Geometry check sheet. Reference: the model listing, model coordinates, mm. Give positions to 0.01 mm unless a question says otherwise; leave off trailing zeros. Write each loop counter-clockwise with the first axis right and the second up, starting at its lowest first coordinate (ties: lowest second). Pieces come first, ordered by that corner, then holes. Notation, with made-up numbers: (80, 69) -> (108, 69) arc R21 ccw to (108, 77) -> close; hole circle Ø10 at (80, -10.5). An arc over 180 degrees is marked (long way). One line per item, written item: value.
from build123d import *

# Parameters (mm, degrees)
F0_W     = 175
F0_H     = 130
F0_R     = 7.5
F1_DEPTH = 15


with BuildPart() as f1:
    # F0 (on Front) → F1 (new body)
    with BuildSketch(Plane.XZ):
        Rectangle(F0_W, F0_H)
        with Locations((-62.5, -40)):
            Circle(F0_R, mode=Mode.SUBTRACT)
        with Locations((-37.5, -40)):
            Circle(F0_R, mode=Mode.SUBTRACT)
        with Locations((-12.5, -40)):
            Circle(F0_R, mode=Mode.SUBTRACT)
        with Locations((12.5, -40)):
            Circle(F0_R, mode=Mode.SUBTRACT)
        with Locations((37.5, -40)):
            Circle(F0_R, mode=Mode.SUBTRACT)
        with Locations((62.5, -40)):
            Circle(F0_R, mode=Mode.SUBTRACT)
        with Locations((-62.5, 0)):
            Circle(F0_R, mode=Mode.SUBTRACT)
        with Locations((-37.5, 0)):
            Circle(F0_R, mode=Mode.SUBTRACT)
        with Locations((-12.5, 0)):
            Circle(F0_R, mode=Mode.SUBTRACT)
        with Locations((-62.5, 40)):
            Circle(F0_R, mode=Mode.SUBTRACT)
        with Locations((-37.5, 40)):
            Circle(F0_R, mode=Mode.SUBTRACT)
        with Locations((-12.5, 40)):
            Circle(F0_R, mode=Mode.SUBTRACT)
        with Locations((12.5, 0)):
            Circle(F0_R, mode=Mode.SUBTRACT)
        with Locations((37.5, 0)):
            Circle(F0_R, mode=Mode.SUBTRACT)
        with Locations((62.5, 0)):
            Circle(F0_R, mode=Mode.SUBTRACT)
        with Locations((12.5, 40)):
            Circle(F0_R, mode=Mode.SUBTRACT)
        with Locations((37.5, 40)):
            Circle(F0_R, mode=Mode.SUBTRACT)
        with Locations((62.5, 40)):
            Circle(F0_R, mode=Mode.SUBTRACT)
    extrude(amount=F1_DEPTH)


solid = f1.part
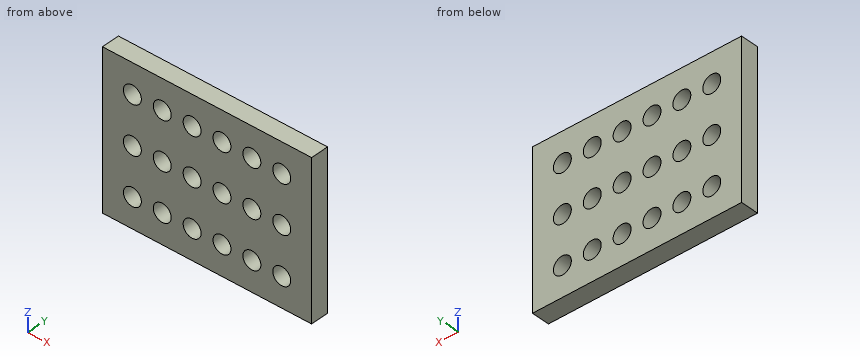
1) Scan lines: probe 1 along Z at (x, y) = (37.5, -4.5); probe 2 along Z at (x, y) = (14.5, -11). Record each from-to range of solid material in increasing order.
Verdict:
probe 1: -65 to -47.5, -32.5 to -7.5, 7.5 to 32.5, 47.5 to 65
probe 2: -65 to -47.23, -32.77 to -7.23, 7.23 to 32.77, 47.23 to 65
2) Sectioned sample at B-B on x = -62.5. Record the cut outline in (y, z), plus the area to 4 significant figures.
Verdict:
outline: (-15, -65) -> (0, -65) -> (0, -47.5) -> (-15, -47.5) -> close; (-15, -32.5) -> (0, -32.5) -> (0, -7.5) -> (-15, -7.5) -> close; (-15, 7.5) -> (0, 7.5) -> (0, 32.5) -> (-15, 32.5) -> close; (-15, 47.5) -> (0, 47.5) -> (0, 65) -> (-15, 65) -> close
area: 1,275 mm^2
3) Depth check by flat-ended pin: pin 1 Ø19.5 at (x, z) = (37.5, 0) entering from -Y. Enter the tip coordinate at first touch or a pass-through.
Verdict:
pin 1: y = -15
4) Sectioned sample at A-A on y = -5.75. Give the number of separate pieces and of enclosed holes in the cut face, plus the area to 3 significant figures.
Verdict:
separate pieces: 1
enclosed holes: 18
area: 19,600 mm^2
5) Sectioned sample at C-C on z = 40. Record the cut outline in (x, y).
Verdict:
outline: (-87.5, -15) -> (-70, -15) -> (-70, 0) -> (-87.5, 0) -> close; (-55, -15) -> (-45, -15) -> (-45, 0) -> (-55, 0) -> close; (-30, -15) -> (-20, -15) -> (-20, 0) -> (-30, 0) -> close; (-5, -15) -> (5, -15) -> (5, 0) -> (-5, 0) -> close; (20, -15) -> (30, -15) -> (30, 0) -> (20, 0) -> close; (45, -15) -> (55, -15) -> (55, 0) -> (45, 0) -> close; (70, -15) -> (87.5, -15) -> (87.5, 0) -> (70, 0) -> close
